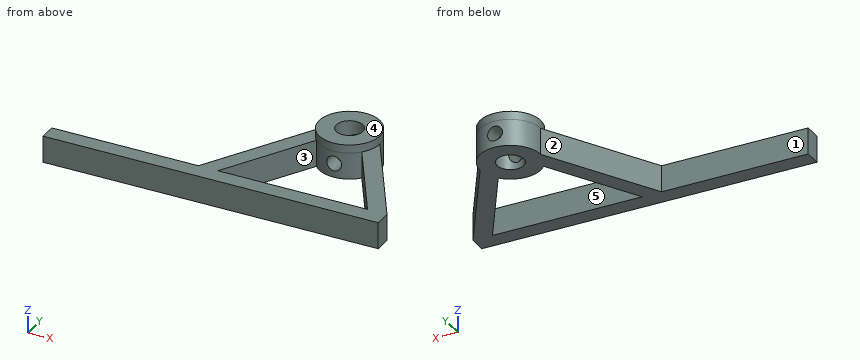
```python
from build123d import *

# Parameters (mm, degrees)
SKETCH1_R               = 3.175
BOSS_EXTRUDE1_DEPTH     = 6.34
CUT_EXTRUDE1_DEPTH      = 4.34
CUT_EXTRUDE1_DEPTH_BACK = 18.34
SKETCH2_R               = 1.775
SKETCH5_R               = 7.235705293
SKETCH5_R_2             = 3.175
BOSS_EXTRUDE2_DEPTH     = 1.96
SKETCH6_W               = 6.34
SKETCH6_H               = 4
BOSS_EXTRUDE3_DEPTH     = 35


with BuildPart() as part:
    # Sketch1 → Boss-Extrude1 (new body)
    with BuildSketch(Plane.XY):
        with BuildLine():
            Line((-7.235705295, 8.319966171), (-22.5, -17.680033829))
            Line((-22.5, -17.680033829), (-22.5, -21.680033829))
            Line((-22.5, -21.680033829), (22.5, -21.680033829))
            Line((22.5, -21.680033829), (22.5, -17.680033829))
            Line((22.5, -17.680033829), (7.235705295, 8.319966171))
            ThreePointArc((7.235705293, 8.319966171), (0, 15.555671463), (-7.235705293, 8.319966171))
        make_face()
        with BuildLine():
            Line((-17.861599202, -17.680033829), (-5.414947439, 3.520614619))
            ThreePointArc((-5.414947439, 3.520614619), (0, 1.084260878), (5.414947439, 3.520614619))
            Line((5.414947439, 3.520614619), (17.861599202, -17.680033829))
            Line((17.861599202, -17.680033829), (-17.861599202, -17.680033829))
        make_face(mode=Mode.SUBTRACT)
        with Locations((0, 8.319966171)):
            Circle(SKETCH1_R, mode=Mode.SUBTRACT)
    extrude(amount=BOSS_EXTRUDE1_DEPTH)

    # Sketch2 → Cut-Extrude1 (cut, two sides: drawn at the far end of the back side and taken through both)
    with BuildSketch(Plane(origin=(0, 14.319966171, 0), x_dir=(1, 0, 0), z_dir=(0, 1, 0)).offset(-CUT_EXTRUDE1_DEPTH_BACK)):
        with Locations(Location((0, -3.35, 0), (0, 0, 90))):
            Circle(SKETCH2_R)
    extrude(amount=CUT_EXTRUDE1_DEPTH + CUT_EXTRUDE1_DEPTH_BACK, mode=Mode.SUBTRACT)

    # Sketch5 → Boss-Extrude2 (add)
    with BuildSketch(Plane.XY.offset(6.34)):
        with Locations((0, 8.319966171)):
            Circle(SKETCH5_R)
        with Locations((0, 8.319966171)):
            Circle(SKETCH5_R_2, mode=Mode.SUBTRACT)
    extrude(amount=BOSS_EXTRUDE2_DEPTH)

    # Sketch6 → Boss-Extrude3 (add)
    with BuildSketch(Plane.ZY.offset(22.5)):
        with Locations((3.17, -19.680033829)):
            Rectangle(SKETCH6_W, SKETCH6_H)
    extrude(amount=BOSS_EXTRUDE3_DEPTH)


solid = part.part
```
Design review of the part built by this model. Coordinates are the model's own, in mm. Face numbers are marked on the shaded views. A direction names the side the tool comes from. Coordinates: 2 decimals unless noted, no trailing zeros. Loops run counter-clockwise (first coordinate to the right, second up) from the corner with the lowest first, then second, coordinate; pieces in that order, holes last.
Q1. We need section C-C on z = 3.35. State the section outline as (x, y) points (3 decimals).
Reported:
outline: (-57.5, -21.68) - (22.5, -21.68) - (22.5, -17.68) - (7.236, 8.32) arc R7.236 ccw to (1.775, 15.335) - (1.775, 10.952) arc R3.175 cw to (1.775, 5.687) - (1.775, 1.305) arc R7.236 ccw to (5.415, 3.521) - (17.862, -17.68) - (-17.862, -17.68) - (-5.415, 3.521) arc R7.236 ccw to (-1.775, 1.305) - (-1.775, 5.687) arc R3.175 cw to (-1.775, 10.952) - (-1.775, 15.335) arc R7.236 ccw to (-7.236, 8.32) - (-22.5, -17.68) - (-57.5, -17.68) - close
Q2. We need section D-D on x = -14.5. State the section outline as (y, z) points.
Reported:
outline: (-21.68, 0) - (-17.68, 0) - (-17.68, 6.34) - (-21.68, 6.34) - close; (-11.95, 0) - (-4.05, 0) - (-4.05, 6.34) - (-11.95, 6.34) - close
Q3. We need section A-A on x = 0. State the section outline as (y, z) points (3 decimals).
Reported:
outline: (-21.68, 0) - (-17.68, 0) - (-17.68, 6.34) - (-21.68, 6.34) - close; (1.084, 0) - (5.145, 0) - (5.145, 1.575) - (1.084, 1.575) - close; (1.084, 5.125) - (5.145, 5.125) - (5.145, 8.3) - (1.084, 8.3) - close; (11.495, 0) - (15.556, 0) - (15.556, 1.575) - (11.495, 1.575) - close; (11.495, 5.125) - (15.556, 5.125) - (15.556, 8.3) - (11.495, 8.3) - close
Q4. To check wall thickness, follow line 1 (Y direction, x = 0, z = 3); line 2 (X direction, y = 2, z = 5.25); line 3 (X direction, y = 8.5, z = 2.25). State the ranges of each line that lie inside material, in increasing order.
Reported:
line 1: y = -21.68 to -17.68
line 2: x = -10.95 to -6.31, -3.52 to 3.52, 6.31 to 10.95
line 3: x = -7.23 to -3.17, 3.17 to 7.23
Q5. For pin 1 (1.5 mm diameter, centred on x = -23.5, z = 6.5, fed in from -Y); pin 2 (2 mm diameter, centred on x = -19.5, y = -14, fed in from +Z); pin 3 (3 mm diameter, centred on x = 0, z = 3.35, fed in from +Y), all flat-tipped, find the tip position at first contact; note any pin that passes through.
Reported:
pin 1: stops at y = -21.68
pin 2: stops at z = 6.34
pin 3: stops at y = -17.68
Q6. We need section B-B on y = -15.5. State the section outline as (x, z) points, and give its area (3 significant figures).
Reported:
outline: (-21.22, 0) - (-16.58, 0) - (-16.58, 6.34) - (-21.22, 6.34) - close; (16.58, 0) - (21.22, 0) - (21.22, 6.34) - (16.58, 6.34) - close
area: 58.8 mm2
Q7. The part is to be moulded in two halves that separate along X. For the marked faces 1, 2 and 3, say which applies: +X half, -X half, draft (parallel to the pull), parting line (faces both ways), or undercut.
Reported:
face 1: draft
face 2: -X half
face 3: undercut
Q8. Tool access review of the marked faces 4 and 5: name each direction out of +Z, -Z, +X, -X, +Y, -Y from which nothing blocks a thin tool from reaching the whole face with its end or side.
Reported:
face 4: +Z, +X, -X, +Y, -Y
face 5: +Z, -Z
